Design review of the part built by this model. Coordinates are the model's own, in mm. Coordinates: 2 decimals unless noted, no trailing zeros. Write each loop counter-clockwise with the first axis right and the second up, starting at its lowest first coordinate (ties: lowest second). Pieces come first, ordered by that corner, then holes. Notation, with made-up numbers: (35, 82.25) -> (79, 82.25) arc R18 ccw to (79, 88.25) -> close; hole circle Ø7 at (61.5, -35.75). An arc over 180 degrees is marked (long way). Answer in a Markdown table with one row per item. Add a question column.
Item 1: To check wall thickness, follow line 1 (Z direction, x = 6, y = 3); line 2 (Z direction, x = 7, y = 10); line 3 (X direction, y = 8.5, z = 31.75). State the ranges of each line that lie inside material, in increasing order.
Item 2: Take a section at A-A, the plane y = 7. Give the number of separate pieces and of enclosed holes in the cut face, and give its area (3 significant figures).
Item 3: Take a section at B-B, the plane z = 19.05. Write out the cut boundary in (x, y), and give its area (3 significant figures).
Item 4: Clearance check with a flat-ended pin moving along its axis: P1, Ø2.5, axis at x = 6.19, z = 6.35, coming from the -Y side (3 decimals). State where the tip first meets the part, or that it passes through.
Item 5: Take a section at C-C, the plane x = 2.75. Write out the cut boundary in (y, z).
Item 6: Draft analysis for pull direction X (two halves, no side actions). For faces 1 (the face through (0, 6, 19)), 2 (the face through (6, 0, 19)), 3 (the face through (12.7, 6, 19)), 4 (the face through (7.86, 6.26, 33.03)), state which applies: released by +X, released by -X, zero draft, split by the parting line, or undercut.
from build123d import *

# Parameters (mm, degrees)
SKETCH1_W                    = 12.7
SKETCH1_H                    = 12.7
BOSS_EXTRUDE1_DEPTH          = 38.1
TAP_DRILL_FOR_M5X0_8_TAP1_D  = 4.2
F_1_8_0_125_DIAMETER_HOLE1_D = 3.175


with BuildPart() as part:
    # Sketch1 → Boss-Extrude1 (new body)
    with BuildSketch(Plane.XY):
        with Locations((6.35, 6.35)):
            Rectangle(SKETCH1_W, SKETCH1_H)
    extrude(amount=BOSS_EXTRUDE1_DEPTH)

    # Tap Drill for M5x0.8 Tap1 (through all)
    with Locations(Plane(origin=(0, 12.7, 0), x_dir=(1, 0, 0), z_dir=(0, 1, 0))):
        with Locations((6.193295447, -6.35), (6.193295447, -31.75)):
            Hole(TAP_DRILL_FOR_M5X0_8_TAP1_D / 2)

    # 1/8 (0.125) Diameter Hole1 (through all)
    with Locations(Plane(origin=(0, 12.7, 0), x_dir=(1, 0, 0), z_dir=(0, 1, 0))):
        with Locations((3.175, -19.05)):
            Hole(F_1_8_0_125_DIAMETER_HOLE1_D / 2)


solid = part.part
Answers:
| question | item | result |
|---|---|---|
| 1 | line 1 | z = 0 to 4.26, 8.44 to 29.66, 33.84 to 38.1 |
| 1 | line 2 | z = 0 to 4.41, 8.29 to 29.81, 33.69 to 38.1 |
| 1 | line 3 | x = 0 to 4.09, 8.29 to 12.7 |
| 2 | separate pieces | 1 |
| 2 | enclosed holes | 3 |
| 2 | area | 448 mm^2 |
| 3 | outline | (0, 0) -> (1.59, 0) -> (1.59, 12.7) -> (0, 12.7) -> close; (4.76, 0) -> (12.7, 0) -> (12.7, 12.7) -> (4.76, 12.7) -> close |
| 3 | area | 121 mm^2 |
| 4 | P1 | passes through |
| 5 | outline | (0, 0) -> (12.7, 0) -> (12.7, 17.52) -> (0, 17.52) -> close; (0, 20.58) -> (12.7, 20.58) -> (12.7, 38.1) -> (0, 38.1) -> close |
| 6 | face 1 | released by -X |
| 6 | face 2 | zero draft |
| 6 | face 3 | released by +X |
| 6 | face 4 | undercut |
